Input: dimensioned drawing with shaded views. Units: mm. Origin: part minimum x, y, z. A direction names the side the tool comes from. Round coordinates to 2 decimals unless told otherwise and drop trailing zeros. Write each loop counter-clockwise with the first axis right and the second up, starting at its lowest first coordinate (ties: lowest second). Pieces come first, ordered by that corner, then holes. Notation, with made-up numbers: (43.25, -20) -> (83.25, -20) arc R19 cw to (83.25, -5) -> close; hole circle Ø6 at (-3.5, 44). An arc over 180 degrees is marked (long way). Use one line per item in the form item = value. Start each with the question number.
1. Reachability of the marked faces 1 and 2 from +Z, -Z, +X, -X, +Y, -Y: full face, straight path, thin tool, end or side. Return the list, or none.
2. Cut plane D-D, the plane y = 5.5. Return the cut outline in (x, z).
3. Cut plane C-C, the plane z = 21.5. Return the cut outline in (x, y).
4. Cut plane A-A, the plane z = 12.7. Return the cut outline in (x, y), plus the area to 3 significant figures.
5. Pin query (flat end, axial travel): pin 1 Ø10 at (x, z) = (31.75, 12.7) entering from -Y; pin 2 Ø1.5 at (x, y) = (51.5, 21.5) entering from +Z. Return the tip coordinate at first contact, or that it passes through.
6. Line query: L1, parallel to Z at x = 31.75, y = 23.85; L2, parallel to X at y = 12.5, z = 3; L3, parallel to X at y = 23.3, z = 12.7. Output: solid intervals per line, ascending.
7. Draft query along X for the marked faces 3, 4 and 5. Return one class per face: pulls with the +X half, pulls with the -X half, needs draft (parallel to the pull), parting line crosses it, or undercut.
8. Cut plane B-B, the plane x = 31.75. Return the cut outline in (y, z).
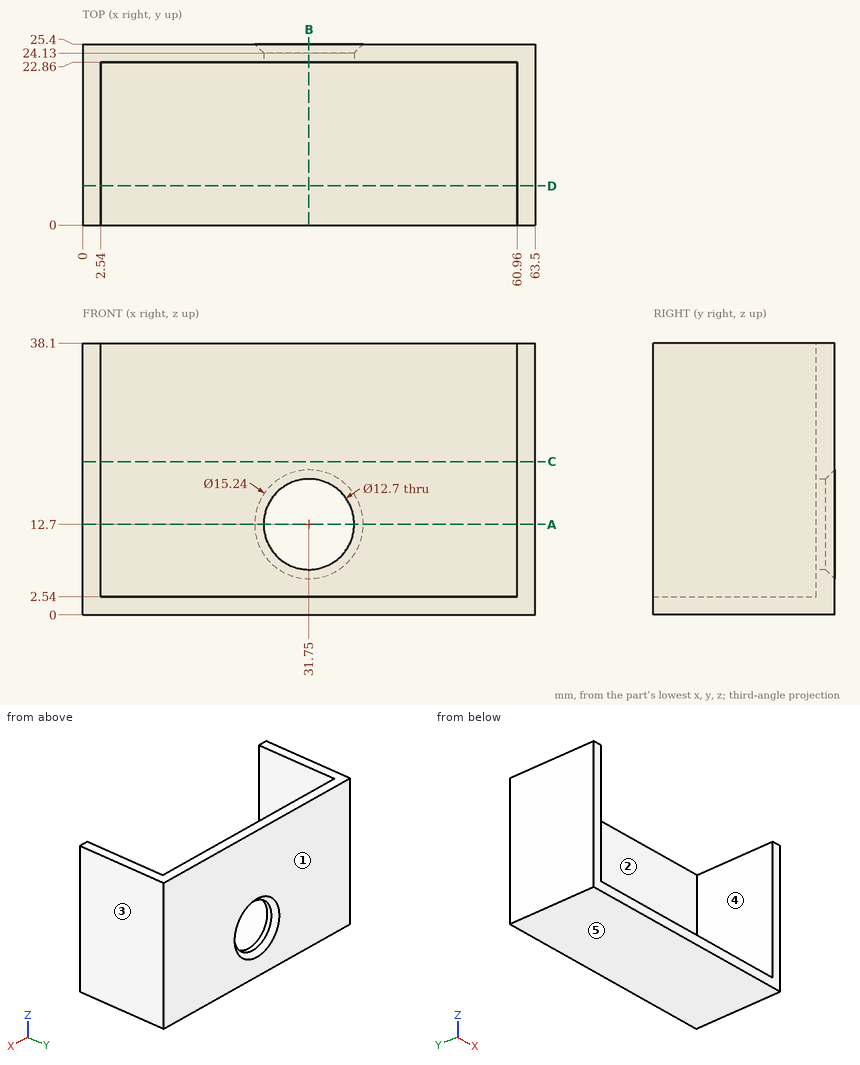
Outcome:
q1.face_1 = +Z, -Z, +X, -X, +Y
q1.face_2 = +Z, -Y
q2.outline = (0, 0) -> (63.5, 0) -> (63.5, 38.1) -> (60.96, 38.1) -> (60.96, 2.54) -> (2.54, 2.54) -> (2.54, 38.1) -> (0, 38.1) -> close
q3.outline = (0, 0) -> (2.54, 0) -> (2.54, 22.86) -> (60.96, 22.86) -> (60.96, 0) -> (63.5, 0) -> (63.5, 25.4) -> (0, 25.4) -> close
q4.outline = (0, 0) -> (2.54, 0) -> (2.54, 22.86) -> (25.4, 22.86) -> (25.4, 24.13) -> (24.13, 25.4) -> (0, 25.4) -> close; (38.1, 22.86) -> (60.96, 22.86) -> (60.96, 0) -> (63.5, 0) -> (63.5, 25.4) -> (39.37, 25.4) -> (38.1, 24.13) -> close
q4.area = 244 mm^2
q5.pin_1 = through
q5.pin_2 = 2.54
q6.L1 = 0 to 6.35, 19.05 to 38.1
q6.L2 = 0 to 2.54, 60.96 to 63.5
q6.L3 = 0 to 25.4, 38.1 to 63.5
q7.face_3 = pulls with the +X half
q7.face_4 = undercut
q7.face_5 = needs draft
q8.outline = (0, 0) -> (25.4, 0) -> (25.4, 5.08) -> (24.13, 6.35) -> (22.86, 6.35) -> (22.86, 2.54) -> (0, 2.54) -> close; (22.86, 19.05) -> (24.13, 19.05) -> (25.4, 20.32) -> (25.4, 38.1) -> (22.86, 38.1) -> close
